from build123d import *

# Parameters (mm, degrees)
SKETCH1_W           = 40
SKETCH1_H           = 20
SKETCH1_R           = 1.9
MAIN_MOUNTING_DEPTH = 4
SKETCH2_W           = 20
SKETCH2_H           = 20
EXTENTION_DEPTH     = 4
SKETCH3_W           = 10
SKETCH3_H           = 6
BOSS_EXTRUDE3_DEPTH = 40.52
SKETCH4_W           = 10
SKETCH4_H           = 5
BOSS_EXTRUDE4_DEPTH = 25
SKETCH5_R           = 1.5
SKETCH5_R_2         = 2.5
CUT_EXTRUDE1_DEPTH  = 62.537227757
SKETCH7_W           = 20
SKETCH7_H           = 14
CUT_EXTRUDE2_DEPTH  = 63.184165187
FILLET1_R           = 10
FILLET2_R           = 5


with BuildPart() as part:
    # Sketch1 → main mounting (new body)
    with BuildSketch(Plane.XY):
        with Locations((0, 10)):
            Rectangle(SKETCH1_W, SKETCH1_H)
        with Locations((-12.5, 15)):
            Circle(SKETCH1_R, mode=Mode.SUBTRACT)
        with Locations((-12.5, 5)):
            Circle(SKETCH1_R, mode=Mode.SUBTRACT)
        with Locations(Location((12.5, 5, 0), (0, 0, 180))):
            Circle(SKETCH1_R, mode=Mode.SUBTRACT)
        with Locations(Location((12.5, 15, 0), (0, 0, 180))):
            Circle(SKETCH1_R, mode=Mode.SUBTRACT)
    extrude(amount=MAIN_MOUNTING_DEPTH)

    # Sketch2 → extention (add)
    with BuildSketch(Plane(origin=(0, 0, 0), x_dir=(-1, 0, 0), z_dir=(0, 0, -1))):
        with Locations((30, 10)):
            Rectangle(SKETCH2_W, SKETCH2_H)
        with Locations((-30, 10)):
            Rectangle(SKETCH2_W, SKETCH2_H)
    extrude(amount=-EXTENTION_DEPTH)

    # Sketch3 → Boss-Extrude3 (add)
    with BuildSketch(Plane.XY.offset(4)):
        with Locations((-35, 3)):
            Rectangle(SKETCH3_W, SKETCH3_H)
        with Locations((35, 3)):
            Rectangle(SKETCH3_W, SKETCH3_H)
    extrude(amount=BOSS_EXTRUDE3_DEPTH)

    # Sketch4 → Boss-Extrude4 (add)
    with BuildSketch(Plane.XZ):
        with Locations((-35, 42.02)):
            Rectangle(SKETCH4_W, SKETCH4_H)
        with Locations((35, 42.02)):
            Rectangle(SKETCH4_W, SKETCH4_H)
    extrude(amount=BOSS_EXTRUDE4_DEPTH)

    # Sketch5 → Cut-Extrude1 (cut, through all)
    with BuildSketch(Plane(origin=(0, 0, 39.52), x_dir=(-1, 0, 0), z_dir=(0, 0, 1))):
        with Locations((35, 19.23)):
            Circle(SKETCH5_R)
        with Locations((35, 5.77)):
            Circle(SKETCH5_R)
        with Locations(Location((-35, 12.5, 0), (0, 0, 180))):
            Circle(SKETCH5_R_2)
        with Locations((35, 12.5)):
            Circle(SKETCH5_R_2)
        with Locations(Location((-35, 5.77, 0), (0, 0, 180))):
            Circle(SKETCH5_R)
        with Locations(Location((-35, 19.23, 0), (0, 0, 180))):
            Circle(SKETCH5_R)
    extrude(amount=CUT_EXTRUDE1_DEPTH, mode=Mode.SUBTRACT)

    # Sketch7 → Cut-Extrude2 (cut, through all)
    with BuildSketch(Plane.XY.offset(4)):
        with Locations((-30, 13)):
            Rectangle(SKETCH7_W, SKETCH7_H)
        with Locations((30, 13)):
            Rectangle(SKETCH7_W, SKETCH7_H)
    extrude(amount=-CUT_EXTRUDE2_DEPTH, mode=Mode.SUBTRACT)

    # Fillet1
    fillet1_edges = [part.edges().sort_by_distance(p)[0] for p in [
        (20, 6, 2),
        (-20, 6, 2),
    ]]
    fillet(fillet1_edges, radius=FILLET1_R)

    # Fillet2
    fillet2_edges = [part.edges().sort_by_distance(p)[0] for p in [
        (40, -25, 42.02),
        (30, -25, 42.02),
        (-40, -25, 42.02),
        (-30, -25, 42.02),
    ]]
    fillet(fillet2_edges, radius=FILLET2_R - 0.0001)  # a hair under: the kernel refuses the full size


solid = part.part
The model under review builds one solid part; all positions refer to its coordinate system, in mm. A direction names the side the tool comes from. Round coordinates to 2 decimals unless told otherwise and drop trailing zeros. Loops run counter-clockwise (first coordinate to the right, second up) from the corner with the lowest first, then second, coordinate; pieces in that order, holes last. Notation, with made-up numbers: M 14,7.25 L 29,7.25 A12 cw 29,13.25 Z; hole C 79.5,-11 d5. An arc over 180 degrees is marked long. Answer as a JSON object with one key per item and string values.
Item 1: Clearance check with flat-ended pins moving along their axes: P1, Ø3.5, axis at x = -12.5, y = 5, coming from the +Z side; P2, Ø5, axis at x = 32.5, y = -10.5, coming from the -Z side; P3, Ø1.5, axis at x = -7, z = 4.5, coming from the -Y side; P4, Ø3, axis at x = 31, z = 11.5, coming from the +Y side. State where each tip first meets the part, or that it passes through.
Check sheet entries:
{"P1": "through", "P2": "z = 39.52", "P3": "y = 0", "P4": "y = 6"}
Item 2: The part is to be moulded in two halves that separate along Y. For faces 1 (the face through (37.31, -13.46, 41.98)), 2 (the face through (-39, -23, 42)), 3 (the face through (-35, 6, 23)), 4 (the face through (-30, 1, 27)), say which applies: +Y half, -Y half, draft (parallel to the pull), parting line (faces both ways), or undercut.
Check sheet entries:
{"face 1": "undercut", "face 2": "-Y half", "face 3": "+Y half", "face 4": "draft"}
Item 3: For line 1 along Y through (x, z) = (12.5, 2.3); line 2 along X through (y, z) = (-5.77, 40.65); line 3 along Y through (x, z) = (-35, 42.85), list the stretches that pass through material, from the lowest coordinate up.
Check sheet entries:
{"line 1": "0 to 3.1, 6.9 to 13.1, 16.9 to 20", "line 2": "-40 to -36.5, -33.5 to -30, 30 to 33.5, 36.5 to 40", "line 3": "-25 to -20.73, -17.73 to -15, -10 to -7.27, -4.27 to 6"}
Item 4: Tool access review of faces 5 (the face through (34.9, -9.5, 39.52)), 6 (the face through (20, 18, 2)), 7 (the face through (31, -23, 42)): name each direction out of +Z, -Z, +X, -X, +Y, -Y from which nothing blocks a thin tool from reaching the whole face with its end or side.
Check sheet entries:
{"face 5": "-Z, +X, -X, -Y", "face 6": "+Z, -Z, +X, +Y", "face 7": "+Z, -Z, -Y"}
Item 5: We need section D-D, the plane y = -5.77. State the section outline as (x, z) points, and give its area (3 significant figures).
Check sheet entries:
{"outline": "M -40,39.52 L -36.5,39.52 L -36.5,44.52 L -40,44.52 Z; M -33.5,39.52 L -30,39.52 L -30,44.52 L -33.5,44.52 Z; M 30,39.52 L 33.5,39.52 L 33.5,44.52 L 30,44.52 Z; M 36.5,39.52 L 40,39.52 L 40,44.52 L 36.5,44.52 Z", "area": "70.0 mm2"}
Item 6: We need section A-A, the plane z = 15. State the section outline as (x, y) points, and give its area (3 significant figures).
Check sheet entries:
{"outline": "M -40,0 L -30,0 L -30,6 L -40,6 Z; M 30,0 L 40,0 L 40,6 L 30,6 Z", "area": "120 mm2"}
Item 7: We need section B-B, the plane y = -12.5. State the section outline as (x, z) points, and give its area (3 significant figures).
Check sheet entries:
{"outline": "M -40,39.52 L -37.5,39.52 L -37.5,44.52 L -40,44.52 Z; M -32.5,39.52 L -30,39.52 L -30,44.52 L -32.5,44.52 Z; M 30,39.52 L 32.5,39.52 L 32.5,44.52 L 30,44.52 Z; M 37.5,39.52 L 40,39.52 L 40,44.52 L 37.5,44.52 Z", "area": "50.0 mm2"}
Item 8: We need section C-C, the plane y = 5. State the section outline as (x, z) points.
Check sheet entries:
{"outline": "M -40,0 L -14.4,0 L -14.4,4 L -30,4 L -30,44.52 L -40,44.52 Z; M -10.6,0 L 10.6,0 L 10.6,4 L -10.6,4 Z; M 14.4,0 L 40,0 L 40,44.52 L 30,44.52 L 30,4 L 14.4,4 Z"}
